Geometry: final body of the model. Coordinates: model frame, mm. Face numbers are marked on the shaded views. Give positions to 0.01 mm unless a question says otherwise; leave off trailing zeros. Write each loop counter-clockwise with the first axis right and the second up, starting at its lowest first coordinate (ties: lowest second). Pieces come first, ordered by that corner, then holes. Notation, with made-up numbers: (84, -34) - (135, -34) arc R12 cw to (135, -24) - close; hole circle Ø1 at (-24, 34.5). An arc over 180 degrees is marked (long way). Return JSON: item names as keys, results as strings.
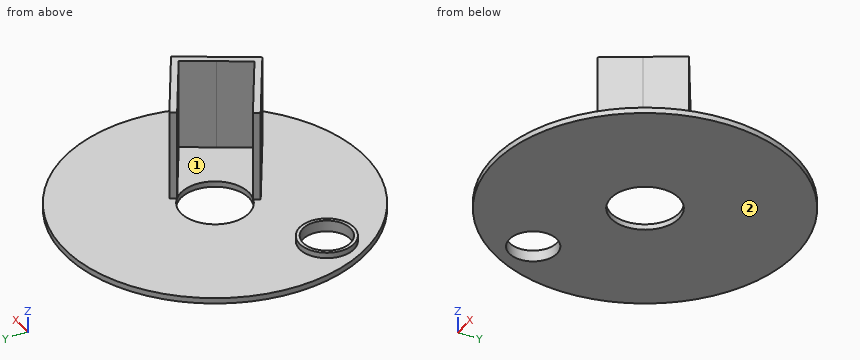
from build123d import *

# Parameters (mm, degrees)
SKETCH1_R           = 66.5
SKETCH1_R_2         = 15
BOSS_EXTRUDE1_DEPTH = 2.5
SKETCH3_R           = 10.5
CUT_EXTRUDE1_DEPTH  = 13.5
BOSS_EXTRUDE2_START = 2.5
SKETCH3_3_R         = 12
SKETCH3_3_R_2       = 10.5
BOSS_EXTRUDE2_DEPTH = 2.5
EXTRUDE_THIN1_DEPTH = 42.5


with BuildPart() as part:
    # Sketch1 → Boss-Extrude1 (new body)
    with BuildSketch(Plane.XY):
        Circle(SKETCH1_R)
        Circle(SKETCH1_R_2, mode=Mode.SUBTRACT)
    extrude(amount=BOSS_EXTRUDE1_DEPTH)

    # Sketch3 → Cut-Extrude1 (cut)
    with BuildSketch(Plane(origin=(-7.303339128, 6.698734651, 2.5), x_dir=(1, 0, 0), z_dir=(0, 0, 1))):
        with Locations((-36.92351869, -31.527257763)):
            Circle(SKETCH3_R)
    extrude(amount=-CUT_EXTRUDE1_DEPTH, mode=Mode.SUBTRACT)

    # Sketch3<3> → Boss-Extrude2 (add)
    with BuildSketch(Plane(origin=(-7.303339128, 6.698734651, 2.5), x_dir=(1, 0, 0), z_dir=(0, 0, 1)).offset(BOSS_EXTRUDE2_START)):
        with Locations((-36.92351869, -31.527257763)):
            Circle(SKETCH3_3_R)
        with Locations((-36.92351869, -31.527257763)):
            Circle(SKETCH3_3_R_2, mode=Mode.SUBTRACT)
    extrude(amount=-BOSS_EXTRUDE2_DEPTH)

    # Sketch13 → Extrude-Thin1 (add)
    with BuildSketch(Plane.XY):
        Polygon((-4.966956498, -13.990954189), (26.209958039, -31.990954189), (33.509958039, -19.346983294), (40.844851528, -6.642575102), (9.667936992, 11.357424898), (11.167336992, 13.954461879), (44.941288509, -5.544938121), (36.106995019, -20.846383294), (27.307595019, -36.08739117), (-6.466356498, -16.58799117), align=None)
    extrude(amount=EXTRUDE_THIN1_DEPTH)


solid = part.part
Q1. Mould query, pull axis Y, two halves, no side actions, for the marked faces 1 and 2. Classes: pulls with the +Y half, pulls with the -Y half, needs draft (parallel to the pull), parting line crosses it, or undercut.
Answer key:
{"face 1": "undercut", "face 2": "needs draft"}
Q2. Material intervals for probe 1 along Y at (x, z) = (0, 1.9); probe 2 along Z at (x, y) = (53, 11.5); probe 3 along X at (y, z) = (-21, 39.5), sorted ascending. Write a range as [from, to].
Answer key:
{"probe 1": "y = [-66.5, -15], [15, 66.5]", "probe 2": "z = [0, 2.5]", "probe 3": "x = [1.18, 7.17], [32.56, 36.02]"}
Q3. Pin query (flat end, axial travel): P1, Ø3, axis at x = -42, y = -47, coming from the -Z side; P2, Ø3, axis at x = 2, y = -33, coming from the +Z side; P3, Ø8, axis at y = -8, z = 10.5, coming from the +X side; P4, Ø5, axis at x = -8, z = 6, coming from the -Y side. Return the tip coordinate at first contact, or that it passes through.
Answer key:
{"P1": "stops at z = 0", "P2": "stops at z = 2.5", "P3": "stops at x = 44.94", "P4": "stops at y = -17.15"}
Q4. Section query B-B, the plane x = -1. Return the cut outline in (y, z).
Answer key:
{"outline": "(-66.49, 0) - (-14.97, 0) - (-14.97, 2.5) - (-16.28, 2.5) - (-16.28, 42.5) - (-19.74, 42.5) - (-19.74, 2.5) - (-66.49, 2.5) - close; (14.97, 0) - (66.49, 0) - (66.49, 2.5) - (14.97, 2.5) - close"}
Q5. Section query A-A, the plane y = 0. Return the cut outline in (x, z).
Answer key:
{"outline": "(-66.5, 0) - (-15, 0) - (-15, 2.5) - (-66.5, 2.5) - close; (15, 0) - (66.5, 0) - (66.5, 2.5) - (35.34, 2.5) - (35.34, 42.5) - (29.34, 42.5) - (29.34, 2.5) - (15, 2.5) - close"}
Q6. Section query C-C, the plane z = 24. Return the cut outline in (x, y), plus the area to 3 significant figures.
Answer key:
{"outline": "(-6.47, -16.59) - (27.31, -36.09) - (44.94, -5.54) - (11.17, 13.95) - (9.67, 11.36) - (40.84, -6.64) - (26.21, -31.99) - (-4.97, -13.99) - close", "area": "322 mm^2"}
Q7. Section query D-D, the plane x = 23.5. Return the cut outline in (y, z), plus the area to 3 significant figures.
Answer key:
{"outline": "(-62.21, 0) - (62.21, 0) - (62.21, 2.5) - (6.83, 2.5) - (6.83, 42.5) - (3.37, 42.5) - (3.37, 2.5) - (-30.43, 2.5) - (-30.43, 42.5) - (-33.89, 42.5) - (-33.89, 2.5) - (-62.21, 2.5) - close", "area": "588 mm^2"}
